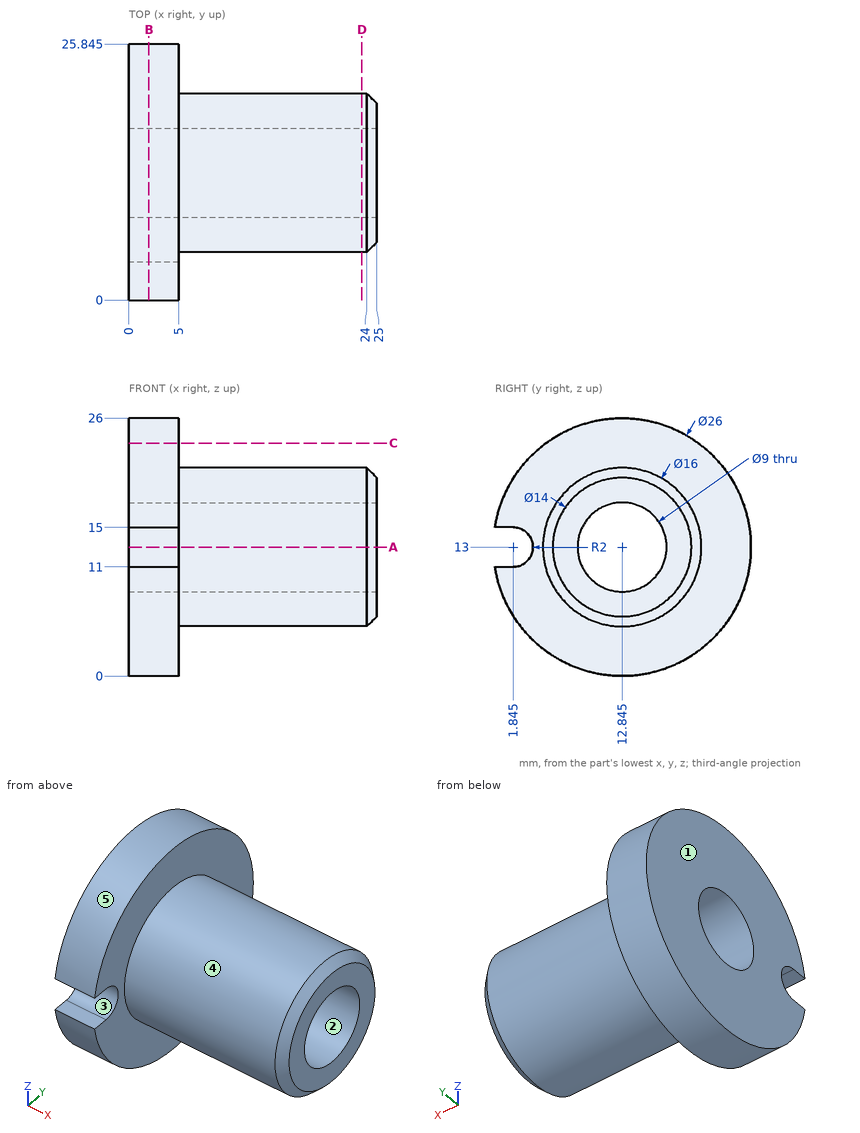
Part print with two shaded views. Sizes in mm from the minimum x, y, z corner. A direction names the side the tool comes from. Coordinates: 2 decimals unless noted, no trailing zeros. Write each loop counter-clockwise with the first axis right and the second up, starting at its lowest first coordinate (ties: lowest second). Pieces come first, ordered by that corner, then holes. Notation, with made-up numbers: M -21.5,78 L 9.5,78 A34 cw 9.5,108 Z; hole C -2,-37.75 d6. An arc over 180 degrees is marked long. Return JSON: item names as keys, results as strings.
Item 1: Probe line 1 (Y direction, x = 8, z = 13) (1 decimal); line 2 (X direction, y = 22.75, z = 7.25); line 3 (Z direction, x = 6.5, y = 13.5). List the from-to ranges inside material, lowest first. Write a range as from..to.
Findings below:
{"line 1": "y = 4.8..8.3, 17.3..20.8", "line 2": "x = 0..5", "line 3": "z = 5.03..8.55, 17.45..20.97"}
Item 2: Which spindle directions (+Z, -Z, +X, -X, +Y, -Y) get a long thin tool onto all of the face, cutting with end or side? Do the marked faces 4 and 5. Say none if no direction does.
Findings below:
{"face 4": "+X", "face 5": "+X, -X"}
Item 3: Slice it at C-C, the plane z = 23.5. Write the cut outline in (x, y).
Findings below:
{"outline": "M 0,5.18 L 5,5.18 L 5,20.51 L 0,20.51 Z"}
Item 4: Drop flat-ended pins along their axis: pin 1 Ø1 at (x, z) = (22.5, 14) entering from -Y; pin 2 Ø2 at (y, z) = (3, 11) entering from +X; pin 3 Ø10 at (x, y) = (22.5, 20.5) entering from +Z. Give the stop position or say it passes through.
Findings below:
{"pin 1": "stops at y = 4.86", "pin 2": "stops at x = 5", "pin 3": "stops at z = 20.55"}
Item 5: Slice it at B-B, the plane x = 2. Write the cut outline in (y, z) (1 decimal).
Findings below:
{"outline": "M 0,11 A13 ccw long 0,15 L 1.8,15 A2 cw 1.8,11 Z; hole C 12.8,13 d9"}
Item 6: Slice it at D-D, the plane x = 23.5. Write the cut outline in (y, z) (1 decimal), and give its area (3 significant figures).
Findings below:
{"outline": "C 12.8,13 d16; hole C 12.8,13 d9", "area": "137 mm2"}
Item 7: Slice it at A-A, the plane z = 13. Write the cut outline in (x, y) (1 decimal).
Findings below:
{"outline": "M 0,3.8 L 5,3.8 L 5,4.8 L 24,4.8 L 25,5.8 L 25,8.3 L 0,8.3 Z; M 0,17.3 L 25,17.3 L 25,19.8 L 24,20.8 L 5,20.8 L 5,25.8 L 0,25.8 Z"}
Item 8: Two-plate mould, pull along Y, no slides. Class the marked faces 1, 2 and 3: +Y half, -Y half, draft (parallel to the pull), parting line (faces both ways), or undercut.
Findings below:
{"face 1": "draft", "face 2": "undercut", "face 3": "-Y half"}
